Source: CAD feature listing. Evaluate the final solid. Frame: model axes, mm. A direction names the side the tool comes from. Give positions to 0.01 mm unless a question says otherwise; leave off trailing zeros. Loops run counter-clockwise (first coordinate to the right, second up) from the corner with the lowest first, then second, coordinate; pieces in that order, holes last. Notation, with made-up numbers: M 5,36.25 L 55,36.25 A16 ccw 55,56.25 Z; hole C -3.5,-36 d2. An arc over 180 degrees is marked long. Put each result on its own line as item: value. Start each with the question number.
```python
from build123d import *

# Parameters (mm, degrees)
SKETCH1_W               = 15.2
SKETCH1_H               = 19.7
EXTRUDE1_DEPTH          = 8
BOSS_EXTRUDE1_DEPTH     = 19.7
SHELL1_T                = -1
SKETCH5_R               = 0.5
EXTRUDE4_DEPTH          = 5
EXTRUDE7_DEPTH          = 10.85
EXTRUDE7_DEPTH_BACK     = 10.85
SKETCH14_W              = 17.7
SKETCH14_H              = 1
CUT_EXTRUDE1_DEPTH      = 6.686379255
CUT_EXTRUDE1_DEPTH_BACK = 5
FILLET1_R               = 0.4
FILLET3_R               = 0.4
FILLET4_R               = 5


with BuildPart() as part:
    # Sketch1 → Extrude1 (new body)
    with BuildSketch(Plane(origin=(0, 0, 0), x_dir=(1, 0, 0), z_dir=(0, 1, 0))):
        Rectangle(SKETCH1_W, SKETCH1_H)
    extrude(amount=EXTRUDE1_DEPTH)

    # Sketch11 → Boss-Extrude1 (add)
    with BuildSketch(Plane.XY.offset(9.85)):
        Polygon((-7.6, 8), (11.063283072, 21.398496459), (18.063283072, 21.398496459), (7.6, 8), align=None)
    extrude(amount=-BOSS_EXTRUDE1_DEPTH)

    # Shell1
    shell1_openings = [part.faces().sort_by_distance(p)[0] for p in [
        (14.563283072, 21.398496459, 0),
        (0, 0, 0),
    ]]
    offset(amount=SHELL1_T, openings=shell1_openings, kind=Kind.INTERSECTION)

    # Sketch5 → Extrude4 (add)
    with BuildSketch(Plane.XZ):
        with Locations((-7.6, 0)):
            Circle(SKETCH5_R)
    extrude(amount=-EXTRUDE4_DEPTH)

    # Sketch9 → Extrude7 (cut, two sides)
    with BuildSketch(Plane.XY) as extrude7_sk:
        Polygon((-7.6, 0), (-8.1, 1.2), (-8.1, 0), align=None)
    extrude(amount=EXTRUDE7_DEPTH, mode=Mode.SUBTRACT)
    extrude(extrude7_sk.sketch, amount=-EXTRUDE7_DEPTH_BACK, mode=Mode.SUBTRACT)

    # Sketch14 → Cut-Extrude1 (cut, two sides)
    with BuildSketch(Plane(origin=(17.4380235, 12.51887437, 0), x_dir=(0, 0, 1), z_dir=(0.812339894, 0.583184274, 0))) as cut_extrude1_sk:
        with Locations((0, -10.43091963)):
            Rectangle(SKETCH14_W, SKETCH14_H)
    extrude(amount=CUT_EXTRUDE1_DEPTH, mode=Mode.SUBTRACT)
    extrude(cut_extrude1_sk.sketch, amount=-CUT_EXTRUDE1_DEPTH_BACK, mode=Mode.SUBTRACT)

    # Fillet1
    fillet1_edges = [part.edges().sort_by_distance(p)[0] for p in [
        (7.6, 8, 0),
        (11.063283072, 21.398496459, -9.35),
        (18.063283072, 21.398496459, 0),
        (12.831641536, 14.699248229, 9.85),
        (14.563283072, 21.398496459, 9.85),
        (1.731641536, 14.699248229, 9.85),
        (1.731641536, 14.699248229, -9.85),
        (14.563283072, 21.398496459, -9.85),
        (12.831641536, 14.699248229, -9.85),
        (-7.6, 8, 0),
        (11.063283072, 21.398496459, 9.35),
        (9.032433338, 19.940535774, -8.85),
        (7.001583604, 18.482575089, 0),
        (9.032433338, 19.940535774, 8.85),
        (-7.6, 4, -9.85),
        (7.6, 4, -9.85),
        (7.6, 4, 9.85),
        (-7.6, 4, 9.85),
    ]]
    fillet(fillet1_edges, radius=FILLET1_R)

    # Fillet3
    fillet3_edges = [part.edges().sort_by_distance(p)[0] for p in [
        (7.584767878, 17.670235196, 0),
    ]]
    fillet(fillet3_edges, radius=FILLET3_R)

    # Fillet4
    fillet4_edges = [part.edges().sort_by_distance(p)[0] for p in [
        (-6.6, 7.48689492, 0),
        (6.6, 8.344203967, 0),
    ]]
    fillet(fillet4_edges, radius=FILLET4_R)


solid = part.part
```
1. Section B-B, the plane z = 0. Output: boundary loops of the cut face in (x, y), plus the area to 3 significant figures.
2. Section A-A, the plane z = 4.75. Output: boundary loops of the cut face in (x, y), plus the area to 3 significant figures.
3. Ray query, line 1 (X direction, y = 2, z = -3.25); line 2 (Z direction, x = -0.25, y = 2); line 3 (X direction, y = 12, z = 2). Return the intervals inside material, ascending.
4. Set-up query: faces 1 (the face through (-6.6, 2, 0)), 2 (the face through (3, 8, 8.85)), 3 (the face through (1.962, 14.716, 9.736)). Return all of +Z, -Z, +X, -X, +Y, -Y with unobstructed straight access to the full face (end or side cutting, diameter ignored); none if empty.
5. Contact query for flat-ended pins moving along their axis: pin 1 (5 mm diameter, centred on x = 0, z = 0, fed in from +Y); pin 2 (3.5 mm diameter, centred on y = 2.5, z = 2, fed in from -X); pin 3 (2 mm diameter, centred on x = 13, z = -1, fed in from +Y). Output: stop coordinate, or through.
6. Pull-direction query (Z, two-part tool) for faces 4 (the face through (6.6, 3, 0)), 5 (the face through (1.962, 14.716, -9.736)), 6 (the face through (6.88, 8.27, 0.12)), 7 (the face through (7.6, 4, 0)); classes: released by +Z, released by -Z, zero draft, split by the parting line, or undercut.
Results found:
1. outline: M -8.1,1.2 L -7.6,0 L -6.6,0 L -6.6,4.92 A5 cw -4.52,8.98 L 7.26,17.44 A0.4 ccw 7.35,18 L 7.23,18.16 A0.4 ccw 6.68,18.25 L -7.43,8.12 A0.4 ccw -7.6,7.79 L -7.6,5 L -8.1,5 Z; M 6.6,0 L 7.6,0 L 7.6,7.86 A0.4 cw 7.68,8.11 L 17.56,20.75 A0.4 ccw 17.24,21.4 L 16.79,21.4 L 7.66,9.7 A5 ccw 6.6,6.62 Z
1. area: 53.1 mm²
2. outline: M -7.6,0 L -6.6,0 L -6.6,4.92 A5 cw -4.52,8.98 L 7.26,17.44 A0.4 ccw 7.35,18 L 7.23,18.16 A0.4 ccw 6.68,18.25 L -7.43,8.12 A0.4 ccw -7.6,7.79 Z; M 6.6,0 L 7.6,0 L 7.6,7.86 A0.4 cw 7.68,8.11 L 17.56,20.75 A0.4 ccw 17.24,21.4 L 16.79,21.4 L 7.66,9.7 A5 ccw 6.6,6.62 Z
2. area: 50.9 mm²
3. line 1: -7.6 to -6.6, 6.6 to 7.6
3. line 2: -9.85 to -8.85, 8.85 to 9.85
3. line 3: -2.03 to -0.31, 9.45 to 10.72
4. face 1: -Y
4. face 2: none
4. face 3: +Z, -X, +Y
5. pin 1: y = 15.25
5. pin 2: x = -8.03
5. pin 3: y = 17.82
6. face 4: undercut
6. face 5: released by -Z
6. face 6: undercut
6. face 7: zero draft
